from build123d import *

# Parameters (mm, degrees)
SKETCH_1_R      = 1.4
SKETCH_1_W      = 15
SKETCH_1_H      = 6
SKETCH_1_W_2    = 6
SKETCH_1_H_2    = 10
EXTRUDE_1_DEPTH = 6


with BuildPart() as part:
    # Эскиз1 → Бобышка-Вытянуть1 (new body)
    with BuildSketch(Plane.XY):
        with BuildLine():
            Line((96.920798757, 2), (96.920798757, 25))
            Line((96.920798757, 25), (96.920798757, 33))
            ThreePointArc((96.920798757, 33), (98.385264851, 36.535533906), (101.920798757, 38))
            Line((101.920798757, 38), (149.389201243, 38))
            Line((149.389201243, 38), (149.389201243, 30))
            Line((149.389201243, 30), (149.389201243, 20.709265489))
            Line((149.389201243, 20.709265489), (143.389201243, 20.709265489))
            Line((143.389201243, 20.709265489), (143.389201243, 10.709265489))
            Line((143.389201243, 10.709265489), (149.389201243, 10.709265489))
            Line((149.389201243, 10.709265489), (149.389201243, -4.290734511))
            Line((149.389201243, -4.290734511), (143.389201243, -4.290734511))
            Line((143.389201243, -4.290734511), (143.389201243, -14.290734511))
            Line((143.389201243, -14.290734511), (149.389201243, -14.290734511))
            Line((149.389201243, -14.290734511), (149.389201243, -30))
            Line((149.389201243, -30), (-144.389201243, -30))
            Line((-144.389201243, -30), (-149.389201243, -25))
            Line((-149.389201243, -25), (-149.389201243, -13))
            Line((-149.389201243, -13), (-128.98858016, -13))
            Line((-128.98858016, -13), (-128.98858016, 7))
            Line((-128.98858016, 7), (-122.58858016, 7))
            Line((-122.58858016, 7), (-122.58858016, 13))
            Line((-122.58858016, 13), (-107.58858016, 13))
            Line((-107.58858016, 13), (-107.58858016, 7))
            Line((-107.58858016, 7), (-101.18858016, 7))
            Line((-101.18858016, 7), (-101.18858016, -13))
            Line((-101.18858016, -13), (24.179035237, -13))
            Line((24.179035237, -13), (24.179035237, 7))
            Line((24.179035237, 7), (31.021419837, 7))
            Line((31.021419837, 7), (31.021419837, 13))
            Line((31.021419837, 13), (46.021419837, 13))
            Line((46.021419837, 13), (46.021419837, 7))
            Line((46.021419837, 7), (52.929060017, 7))
            Line((52.929060017, 7), (52.929060017, -13))
            Line((52.929060017, -13), (81.920798757, -13))
            ThreePointArc((81.920798757, -13), (92.527400475, -8.606601718), (96.920798757, 2))
        make_face()
        with Locations((104.970798757, -19)):
            Circle(SKETCH_1_R, mode=Mode.SUBTRACT)
        with Locations((104.970798757, 25)):
            Circle(SKETCH_1_R, mode=Mode.SUBTRACT)
        with Locations((111.920798757, 3.209265489)):
            Circle(SKETCH_1_R, mode=Mode.SUBTRACT)
        with Locations((146.389201243, 3.209265489)):
            Circle(SKETCH_1_R, mode=Mode.SUBTRACT)
        with Locations((-128.98858016, -19)):
            Circle(SKETCH_1_R, mode=Mode.SUBTRACT)
        with Locations((-28.18858016, -19)):
            Circle(SKETCH_1_R, mode=Mode.SUBTRACT)
        with Locations((62.61141984, -19)):
            Circle(SKETCH_1_R, mode=Mode.SUBTRACT)
        with Locations((129.420798757, -19)):
            Rectangle(SKETCH_1_W, SKETCH_1_H, mode=Mode.SUBTRACT)
        with Locations((111.920798757, 15.709265489)):
            Rectangle(SKETCH_1_W_2, SKETCH_1_H_2, mode=Mode.SUBTRACT)
        with Locations((111.920798757, -9.290734511)):
            Rectangle(SKETCH_1_W_2, SKETCH_1_H_2, mode=Mode.SUBTRACT)
        with Locations((129.155798757, 33)):
            Rectangle(SKETCH_1_W, SKETCH_1_H, mode=Mode.SUBTRACT)
    extrude(amount=EXTRUDE_1_DEPTH)


solid = part.part
Design review of the part built by this model. Coordinates are the model's own, in mm. A direction names the side the tool comes from. Give positions to 0.01 mm unless a question says otherwise; leave off trailing zeros. Loops run counter-clockwise (first coordinate to the right, second up) from the corner with the lowest first, then second, coordinate; pieces in that order, holes last. Notation, with made-up numbers: M 81,-36.75 L 85,-36.75 A10 cw 85,-21.75 Z; hole C -1,80 d11. An arc over 180 degrees is marked long. Answer as a JSON object with one key per item and string values.
Item 1: We need section A-A (x = -79). State the section outline as (y, z) points, and give its area (3 significant figures).
Output values:
{"outline": "M -30,0 L -13,0 L -13,6 L -30,6 Z", "area": "102 mm2"}
Item 2: Machinability: for faces 5 (the face through (-122.589, 10, 3)), 6 (the face through (-149.389, -19, 3)), 7 (the face through (143.389, 16, 3)), 8 (the face through (112, 10.709, 3)), 9 (the face through (67, -13, 3)), which of the approach directions +Z, -Z, +X, -X, +Y, -Y give a long, thin tool a straight path to every point of the face, cutting with its end or side? Answer none if there is none.
Output values:
{"face 5": "+Z, -Z, -X, +Y", "face 6": "+Z, -Z, -X, +Y, -Y", "face 7": "+Z, -Z, +X", "face 8": "+Z, -Z", "face 9": "+Z, -Z, +Y"}
Item 3: For P1, Ø3, axis at y = 14.5, z = 1.5, coming from the +X side; P2, Ø3.5, axis at x = -28.19, y = -19, coming from the +Z side; P3, Ø3, axis at y = 1.5, z = 4, coming from the -X side; P4, Ø1.8, axis at y = 33, z = 3.5, coming from the -X side, all flat-tipped, find the tip position at first contact; note any pin that passes through.
Output values:
{"P1": "stops at x = 143.39", "P2": "stops at z = 6", "P3": "stops at x = -128.99", "P4": "stops at x = 96.92"}
Item 4: We need section B-B (z = 4.05). Count the separate pieces of the cut face and the enclosed holes in it, and give its area (3 significant figures).
Output values:
{"separate pieces": "1", "enclosed holes": "11", "area": "8,630 mm2"}
Item 5: Wall thickness on line 1 along X through (y, z) = (8, 0.3); line 2 along Y through (x, z) = (74.5, 0.5); line 3 along X through (y, z) = (-21, 3.65): over which ranges is each line inside the solid? List them lowest first.
Output values:
{"line 1": "x = -122.59 to -107.59, 31.02 to 46.02, 96.92 to 149.39", "line 2": "y = -30 to -13", "line 3": "x = -149.39 to 121.92, 136.92 to 149.39"}
Item 6: Mouldability with a two-part tool opening along X and no side actions: class faces 1 (the face through (98.35, 36.5, 2.96)), 2 (the face through (35, -11, 6)), 3 (the face through (121.656, 33, 3)), 4 (the face through (149.389, 29, 3)) as pulls with the +X half, pulls with the -X half, needs draft (parallel to the pull), parting line crosses it, or undercut.
Output values:
{"face 1": "pulls with the -X half", "face 2": "needs draft", "face 3": "undercut", "face 4": "pulls with the +X half"}
